Design review of the part built by this model. Coordinates are the model's own, in mm. A direction names the side the tool comes from. Give positions to 0.01 mm unless a question says otherwise; leave off trailing zeros. Loops run counter-clockwise (first coordinate to the right, second up) from the corner with the lowest first, then second, coordinate; pieces in that order, holes last. Notation, with made-up numbers: (21, -25.75) - (58, -25.75) arc R19 ccw to (58, 2.25) - close; hole circle Ø2 at (-18, 26). An arc over 180 degrees is marked (long way). Write each question's results on one line, items separated by ' | '.
from build123d import *

# Parameters (mm, degrees)
ESQUISSE1_R             = 2.5
ESQUISSE1_R_2           = 3
ESQUISSE1_W             = 40
ESQUISSE1_H             = 8
BOSS_EXTRU_1_DEPTH      = 6
ESQUISSE2_R             = 2.5
BOSS_EXTRU_2_DEPTH      = 8
CONG_2_R                = 2
ENL_V_MAT_EXTRU_1_DEPTH = 4
ENL_V_START             = -10
ENL_V_MAT_EXTRU_4_DEPTH = 10


with BuildPart() as part:
    # Esquisse1 → Boss.-Extru.1 (new body)
    with BuildSketch(Plane.XY):
        with BuildLine():
            Line((90, -15), (-90, -15))
            ThreePointArc((-90, -15), (-105, 0), (-90, 15))
            Line((-90, 15), (90, 15))
            ThreePointArc((90, 15), (105, 0), (90, -15))
        make_face()
        with Locations((99, 0)):
            Circle(ESQUISSE1_R, mode=Mode.SUBTRACT)
        with Locations(Location((-90, 0, 0), (0, 0, 180))):
            Circle(ESQUISSE1_R_2, mode=Mode.SUBTRACT)
        with BuildLine():
            Line((15, -2.5), (-75, -2.5))
            ThreePointArc((-75, -2.5), (-77.5, 0), (-75, 2.5))
            Line((-75, 2.5), (15, 2.5))
            ThreePointArc((15, 2.5), (17.5, 0), (15, -2.5))
        make_face(mode=Mode.SUBTRACT)
        with Locations((60, 0)):
            Rectangle(ESQUISSE1_W, ESQUISSE1_H, mode=Mode.SUBTRACT)
    extrude(amount=BOSS_EXTRU_1_DEPTH)

    # Esquisse2 → Boss.-Extru.2 (add)
    with BuildSketch(Plane(origin=(40, 0, 0), x_dir=(0, 0, -1), z_dir=(1, 0, 0))):
        Polygon((-16, 5), (-16, -5), (-6, -15), (-6, -5), (-6, 5), (-6, 15), align=None)
        with Locations((-11, 0)):
            Circle(ESQUISSE2_R, mode=Mode.SUBTRACT)
    extrude(amount=-BOSS_EXTRU_2_DEPTH)

    # Congé2
    cong_2_edges = [part.edges().sort_by_distance(p)[0] for p in [
        (40, 9.5, 6),
        (40, -9.5, 6),
    ]]
    fillet(cong_2_edges, radius=CONG_2_R)

    # Esquisse3 → Enlèv. mat.-Extru.1 (cut)
    with BuildSketch(Plane.ZY.offset(-32)):
        Polygon((11, 4), (14.464101615, 2), (14.464101615, -2), (11, -4), (7.535898385, -2), (7.535898385, 2), align=None)
    extrude(amount=-ENL_V_MAT_EXTRU_1_DEPTH, mode=Mode.SUBTRACT)

    # Esquisse4 → Enlèv. mat.-Extru.4 (cut)
    with BuildSketch(Plane.XY.offset(6).offset(ENL_V_START)):
        with BuildLine():
            ThreePointArc((-105, -2.6e-08), (-103.148050285, -2.771638603), (-99.878679656, -2.121320344))
            Line((-99.878679656, -2.121320344), (-104.121320344, 2.121320344))
            ThreePointArc((-104.121320344, 2.121320344), (-104.771638603, 1.148050285), (-105, -2.6e-08))
        make_face()
        with BuildLine():
            Line((-104.121320344, 2.121320344), (-99.878679656, -2.121320344))
            ThreePointArc((-99.878679656, -2.121320344), (-99.228361402, -1.148050297), (-99, 0))
            ThreePointArc((-99, 0), (-100.851949703, 2.771638598), (-104.121320344, 2.121320344))
        make_face()
        with BuildLine():
            ThreePointArc((-105, -2.6e-08), (-104.771638603, 1.148050285), (-104.121320344, 2.121320344))
            Line((-104.121320344, 2.121320344), (-104.94364809, 1.298992597))
            ThreePointArc((-104.94364809, 1.298992597), (-104.985905401, 0.650107152), (-105, -2.6e-08))
        make_face()
        with BuildLine():
            Line((-103.750652313, -5.993293), (-99.878679656, -2.121320344))
            ThreePointArc((-99.878679656, -2.121320344), (-103.148050285, -2.771638603), (-105, -2.6e-08))
            ThreePointArc((-105, -2.6e-08), (-104.684341738, -3.061063171), (-103.750652313, -5.993293))
        make_face()
        with BuildLine():
            ThreePointArc((-105, -2.6e-08), (-103.148050285, -2.771638603), (-99.878679656, -2.121320344))
            Line((-99.878679656, -2.121320344), (-104.121320344, 2.121320344))
            ThreePointArc((-104.121320344, 2.121320344), (-104.771638603, 1.148050285), (-105, -2.6e-08))
        make_face()
        with BuildLine():
            Line((-104.121320344, 2.121320344), (-99.878679656, -2.121320344))
            ThreePointArc((-99.878679656, -2.121320344), (-99.228361402, -1.148050297), (-99, 0))
            ThreePointArc((-99, 0), (-100.851949703, 2.771638598), (-104.121320344, 2.121320344))
        make_face()
    extrude(amount=ENL_V_MAT_EXTRU_4_DEPTH, mode=Mode.SUBTRACT)


solid = part.part
(1) Wall thickness on line 1 along Y through (x, z) = (-44, 3.25); line 2 along Y through (x, z) = (50, 2.5); line 3 along Z through (x, y) = (-17, -5): over which ranges is each line inside the solid? List them lowest first. Write a range as from..to.
Answers below:
line 1: -15..-2.5, 2.5..15 | line 2: -15..-4, 4..15 | line 3: 0..6
(2) Tool access review of faces 1 (the flat face through (33.972, 3.014, 12.708)), 2 (the flat face through (-36, 4, 6)), 3 (the flat face through (80, 0, 3)): name each direction out of +Z, -Z, +X, -X, +Y, -Y from which nothing blocks a thin tool from reaching the whole face with its end or side.
Answers below:
face 1: -X | face 2: +Z, -X, +Y, -Y | face 3: +Z, -Z
(3) Insertion check: P1, Ø10, axis at x = -19.5, y = 4, coming from the -Z side; P2, Ø5.5, axis at y = 2, z = 12.5, coming from the -X side; P3, Ø6, axis at y = 6.5, z = 12.5, coming from the +X side. Each pin has a flat end and moves straight along its axis. Give the tip position at first contact, or say it passes through.
Answers below:
P1: z = 0 | P2: x = 32 | P3: x = 40
(4) Take a section at B-B on y = -9. Give the boundary of the cut face in (x, z), plus the area to 3 significant figures.
Answers below:
outline: (-102, 0) - (102, 0) - (102, 6) - (42, 6) arc R2 cw to (40, 8) - (40, 12) - (32, 12) - (32, 6) - (-102, 6) - close | area: 1,270 mm2
(5) Draft analysis for pull direction Z (two halves, no side actions). For faces 4 (the cylindrical face through (97, -1.5, 3)), 5 (the flat face through (33.972, -3.014, 9.292)), 6 (the flat face through (36, -10, 11)), state which applies: pulls with the +Z half, pulls with the -Z half, needs draft (parallel to the pull), parting line crosses it, or undercut.
Answers below:
face 4: needs draft | face 5: undercut | face 6: pulls with the +Z half
(6) Take a section at D-D on x = -82. Give the boundary of the cut face in (y, z), plus the area to 3 significant figures.
Answers below:
outline: (-15, 0) - (15, 0) - (15, 6) - (-15, 6) - close | area: 180 mm2
(7) Take a section at C-C on x = 76. Give the boundary of the cut face in (y, z).
Answers below:
outline: (-15, 0) - (-4, 0) - (-4, 6) - (-15, 6) - close; (4, 0) - (15, 0) - (15, 6) - (4, 6) - close
(8) Take a section at A-A on x = -52. Give the boundary of the cut face in (y, z), plus the area to 3 significant figures.
Answers below:
outline: (-15, 0) - (-2.5, 0) - (-2.5, 6) - (-15, 6) - close; (2.5, 0) - (15, 0) - (15, 6) - (2.5, 6) - close | area: 150 mm2
